Work out the finished part from the listing and answer in its coordinate system (mm). Face numbers are marked on the shaded views. Coordinates: 2 decimals unless noted, no trailing zeros. Order: outer loops, then holes, each group sorted by start corner. A loop starts at its lowest first (then second) coordinate and runs counter-clockwise, first axis right, second up.
```python
from build123d import *

# Parameters (mm, degrees)
F0_R     = 11
F1_DEPTH = 6


with BuildPart() as f1:
    # F0 (on Top) → F1 (new body)
    with BuildSketch(Plane.XY):
        with BuildLine():
            ThreePointArc((8.291562, -12.5), (0, 15), (-8.291562, -12.5))
            ThreePointArc((-8.291562, -12.5), (-13.21691, -17.906814), (-15, -25))
            ThreePointArc((-15, -25), (-13.21691, -32.093186), (-8.291562, -37.5))
            ThreePointArc((-8.291562, -37.5), (0, -65), (8.291562, -37.5))
            ThreePointArc((8.291562, -37.5), (13.21691, -32.093186), (15, -25))
            ThreePointArc((15, -25), (13.21691, -17.906814), (8.291562, -12.5))
        make_face()
        with Locations((0, -50)):
            Circle(F0_R, mode=Mode.SUBTRACT)
        with BuildLine():
            ThreePointArc((-11, -25), (0, -14), (11, -25))
            ThreePointArc((11, -25), (0, -36), (-11, -25))
        make_face(mode=Mode.SUBTRACT)
        Circle(F0_R, mode=Mode.SUBTRACT)
    extrude(amount=F1_DEPTH)


solid = f1.part
```
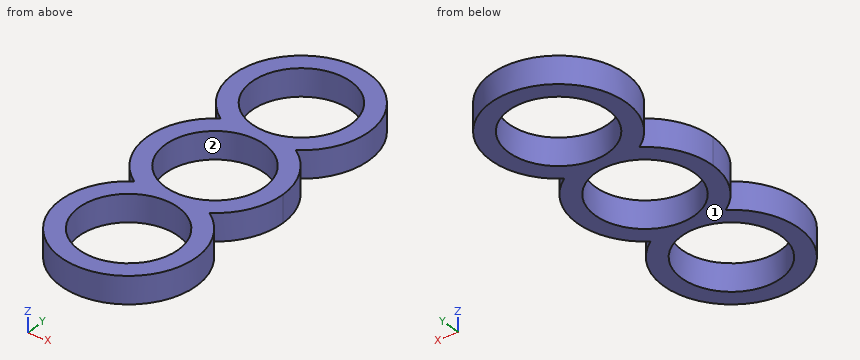
1. The part is cut by section B-B (z = 2.9). Determine the outline of the cut face in (x, y), plus the area to 3 significant figures.
2. The part is cut by section C-C (y = -50). Determine the outline of the cut face in (x, z), plus the area to 3 significant figures.
3. The part is cut by section A-A (x = 0). Determine the outline of the cut face in (y, z).
4. Flat-ended cylindrical pins translate along their axes: pin 1 (3 mm diameter, centred on x = -6, z = 1, fed in from +Y); pin 2 (1.5 mm diameter, centred on y = -35.5, z = 1, fed in from -X); pin 3 (2 mm diameter, centred on y = -23.5, z = 3, fed in from +X). Find the tip coordinate at first contact, or state that the pin passes through.
5. The part is cut by section D-D (y = -21). Determine the outline of the cut face in (x, z).
6. The mould has two halves that part along X. Classify the marked faces 1 and 2: released by +X, released by -X, zero draft, split by the parting line, or undercut.
7. Consider probe 1 along Y at (x, z) = (0, 4.1); probe 2 along Y at (x, z) = (-1.5, 2.45); probe 3 along X at (y, z) = (-25, 1.95). Determine where each line is inside the solid, lowest interval first.
Worked out:
1. outline: (-8.29, -37.5) arc R15 ccw (long way) to (8.29, -37.5) arc R15 ccw to (8.29, -12.5) arc R15 ccw (long way) to (-8.29, -12.5) arc R15 ccw to start; hole circle Ø22 at (0, -50); hole circle Ø22 at (0, -25); hole circle Ø22 at (0, 0)
1. area: 868 mm2
2. outline: (-15, 0) - (-11, 0) - (-11, 6) - (-15, 6) - close; (11, 0) - (15, 0) - (15, 6) - (11, 6) - close
2. area: 48.0 mm2
3. outline: (-65, 0) - (-61, 0) - (-61, 6) - (-65, 6) - close; (-39, 0) - (-36, 0) - (-36, 6) - (-39, 6) - close; (-14, 0) - (-11, 0) - (-11, 6) - (-14, 6) - close; (11, 0) - (15, 0) - (15, 6) - (11, 6) - close
4. pin 1: stops at y = 14.31
4. pin 2: stops at x = -11.4
4. pin 3: stops at x = 14.99
5. outline: (-14.46, 0) - (-10.25, 0) - (-10.25, 6) - (-14.46, 6) - close; (10.25, 0) - (14.46, 0) - (14.46, 6) - (10.25, 6) - close
6. face 1: zero draft
6. face 2: undercut
7. probe 1: y = -65 to -61, -39 to -36, -14 to -11, 11 to 15
7. probe 2: y = -64.92 to -60.9, -39.1 to -35.9, -14.1 to -10.9, 10.9 to 14.92
7. probe 3: x = -15 to -11, 11 to 15
